Source: CAD feature listing. Evaluate the final solid. Frame: model axes, mm. A direction names the side the tool comes from. Give positions to 0.01 mm unless a question says otherwise; leave off trailing zeros. Order: outer loops, then holes, each group sorted by start corner. A loop starts at its lowest first (then second) coordinate and runs counter-clockwise, first axis right, second up. Notation, with made-up numbers: (-26, 4) -> (-9, 4) arc R25 ccw to (-9, 37) -> close; hole circle Ø3 at (52, -27). An arc over 180 degrees is marked (long way). Use one line per item in the form item = value. Start each with the question number.
from build123d import *

# Parameters (mm, degrees)
SKETCH1_W           = 175
SKETCH1_H           = 125
BOSS_EXTRUDE1_DEPTH = 35
SKETCH2_W           = 175
SKETCH2_H           = 125
BOSS_EXTRUDE2_DEPTH = 4
SKETCH3_R           = 2.045
CUT_EXTRUDE1_DEPTH  = 6
SKETCH4_R           = 3.81
CUT_EXTRUDE2_DEPTH  = 10
SKETCH5_R           = 6
SKETCH5_R_2         = 6.35
CUT_EXTRUDE3_DEPTH  = 10


with BuildPart() as part:
    # Sketch1 → Boss-Extrude1 (new body)
    with BuildSketch(Plane.XY):
        with Locations((-87.5, 62.5)):
            Rectangle(SKETCH1_W, SKETCH1_H)
        Polygon((-93.5, 121), (-164, 121), (-164, 114), (-171, 114), (-171, 11), (-164, 11), (-164, 4), (-93.5, 4), (-93.5, 11), (-81.5, 11), (-81.5, 4), (-11, 4), (-11, 11), (-4, 11), (-4, 114), (-11, 114), (-11, 121), (-81.5, 121), (-81.5, 114), (-93.5, 114), align=None, mode=Mode.SUBTRACT)
    extrude(amount=BOSS_EXTRUDE1_DEPTH)

    # Sketch2 → Boss-Extrude2 (add)
    with BuildSketch(Plane.XY.offset(35)):
        with Locations((-87.5, 62.5)):
            Rectangle(SKETCH2_W, SKETCH2_H)
    extrude(amount=BOSS_EXTRUDE2_DEPTH)

    # Sketch3 → Cut-Extrude1 (cut)
    with BuildSketch(Plane(origin=(0, 0, 0), x_dir=(-1, 0, 0), z_dir=(0, 0, -1))):
        with Locations((6, 119)):
            Circle(SKETCH3_R)
        with Locations((87.5, 119)):
            Circle(SKETCH3_R)
        with Locations((169, 119)):
            Circle(SKETCH3_R)
        with Locations((169, 6)):
            Circle(SKETCH3_R)
        with Locations((87.5, 6)):
            Circle(SKETCH3_R)
        with Locations((6, 6)):
            Circle(SKETCH3_R)
    extrude(amount=-CUT_EXTRUDE1_DEPTH, mode=Mode.SUBTRACT)

    # Sketch4 → Cut-Extrude2 (cut)
    with BuildSketch(Plane(origin=(0, 0, 0), x_dir=(0, 0, -1), z_dir=(1, 0, 0))):
        with Locations((-19.5, 87.5)):
            Circle(SKETCH4_R)
        with Locations((-19.5, 62.5)):
            Circle(SKETCH4_R)
        with Locations((-19.5, 37.5)):
            Circle(SKETCH4_R)
    extrude(amount=-CUT_EXTRUDE2_DEPTH, mode=Mode.SUBTRACT)

    # Sketch5 → Cut-Extrude3 (cut)
    with BuildSketch(Plane.ZY.offset(175)):
        with Locations((19.5, 100)):
            Circle(SKETCH5_R)
        with Locations((19.5, 75)):
            Circle(SKETCH5_R_2)
    extrude(amount=-CUT_EXTRUDE3_DEPTH, mode=Mode.SUBTRACT)


solid = part.part
1) Draft query along Y for faces 4 (the face through (-89, 125, 19)), 5 (the face through (-1.97, 34.12, 17.74)), 6 (the face through (-89, 63, 39)). Return one class per face: +Y half, -Y half, draft (parallel to the pull), parting line (faces both ways), or undercut.
2) Cut plane D-D, the plane y = 119. Return the cut outline in (x, z) (3 decimals), plus the area to 3 significant figures.
3) Cut plane C-C, the plane z = 29.5. Return the cut outline in (x, y).
4) Pin query (flat end, axial travel): pin 1 (6 mm diameter, centred on x = -89, z = 17, fed in from -Y); pin 2 (1.2 mm diameter, centred on x = -6.5, y = 119, fed in from -Z); pin 3 (8 mm diameter, centred on x = -80, y = 52, fed in from -Z); pin 4 (11 mm diameter, centred on y = 100, z = 19.5, fed in from -X). Return the tip coordinate at first contact, or that it passes through.
5) Cut plane A-A, the plane y = 37.5. Return the cut outline in (x, z).
6) Material intervals for probe 1 along X at (y, z) = (7.5, 17); probe 2 along Y at (x, z) = (-169, 1.6) (3 decimals); probe 3 along Y at (x, z) = (-19, 4), sorted ascending.
7) Cut plane B-B, the plane x = -87.5. Return the cut outline in (y, z) (3 decimals).
8) Reachability of faces 1 (the face through (-173.03, 68.8, 18.12)), 2 (the face through (-88, 123, 0)), 3 (the face through (-47, 4, 17)) from +Z, -Z, +X, -X, +Y, -Y: full face, straight path, thin tool, end or side. Return the list, or none.
Output values:
q1.face_4 = +Y half
q1.face_5 = undercut
q1.face_6 = draft
q2.outline = (-175, 0) -> (-171.045, 0) -> (-171.045, 6) -> (-166.955, 6) -> (-166.955, 0) -> (-164, 0) -> (-164, 35) -> (-93.5, 35) -> (-93.5, 0) -> (-89.545, 0) -> (-89.545, 6) -> (-85.455, 6) -> (-85.455, 0) -> (-81.5, 0) -> (-81.5, 35) -> (-11, 35) -> (-11, 0) -> (-8.045, 0) -> (-8.045, 6) -> (-3.955, 6) -> (-3.955, 0) -> (0, 0) -> (0, 39) -> (-175, 39) -> close
q2.area = 1,820 mm^2
q3.outline = (-175, 0) -> (0, 0) -> (0, 125) -> (-175, 125) -> close; hole (-171, 11) -> (-164, 11) -> (-164, 4) -> (-93.5, 4) -> (-93.5, 11) -> (-81.5, 11) -> (-81.5, 4) -> (-11, 4) -> (-11, 11) -> (-4, 11) -> (-4, 114) -> (-11, 114) -> (-11, 121) -> (-81.5, 121) -> (-81.5, 114) -> (-93.5, 114) -> (-93.5, 121) -> (-164, 121) -> (-164, 114) -> (-171, 114) -> close
q4.pin_1 = 0
q4.pin_2 = 6
q4.pin_3 = 35
q4.pin_4 = -4
q5.outline = (-175, 0) -> (-171, 0) -> (-171, 35) -> (-4, 35) -> (-4, 23.31) -> (0, 23.31) -> (0, 39) -> (-175, 39) -> close; (-4, 0) -> (0, 0) -> (0, 15.69) -> (-4, 15.69) -> close
q6.probe_1 = -175 to -164, -93.5 to -81.5, -11 to 0
q6.probe_2 = 0 to 3.955, 8.045 to 11, 114 to 116.955, 121.045 to 125
q6.probe_3 = 0 to 4, 121 to 125
q7.outline = (0, 0) -> (3.955, 0) -> (3.955, 6) -> (8.045, 6) -> (8.045, 0) -> (11, 0) -> (11, 35) -> (114, 35) -> (114, 0) -> (116.955, 0) -> (116.955, 6) -> (121.045, 6) -> (121.045, 0) -> (125, 0) -> (125, 39) -> (0, 39) -> close
q8.face_1 = -X
q8.face_2 = -Z, +X, -X, +Y, -Y
q8.face_3 = -Z
